```python
from build123d import *

# Parameters (mm, degrees)
F0_R     = 5.334
F0_R_2   = 1.778
F1_DEPTH = 3.81
F2_R     = 3.048
F3_DEPTH = 3.302


with BuildPart() as f1:
    # F0 (on Top) → F1 (new body)
    with BuildSketch(Plane.XY):
        Circle(F0_R)
        Circle(F0_R_2, mode=Mode.SUBTRACT)
        Circle(F0_R_2)
    extrude(amount=F1_DEPTH)

    # F2
    f2_edges = [f1.edges().sort_by_distance(p)[0] for p in [
        (-5.334, 0, 3.81),
    ]]
    fillet(f2_edges, radius=F2_R)

    # F0 (on Top) → F3 (cut)
    with BuildSketch(Plane.XY):
        Circle(F0_R_2)
    extrude(amount=F3_DEPTH, mode=Mode.SUBTRACT)


solid = f1.part
```
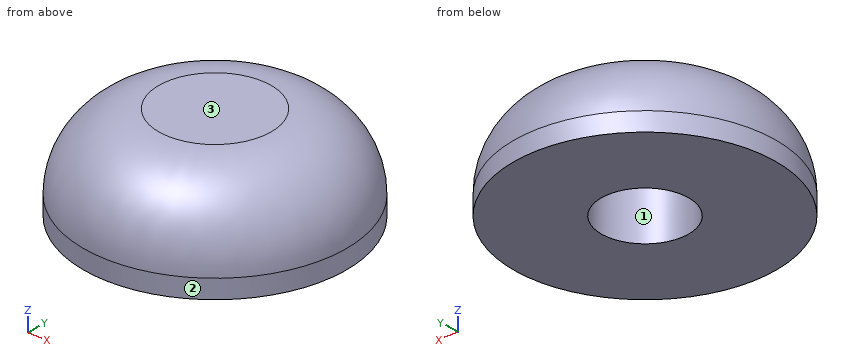
Geometry: final body of the model. Coordinates: model frame, mm. Face numbers are marked on the shaded views. Round coordinates to 2 decimals unless told otherwise and drop trailing zeros.
Item 1: Material intervals for L1, parallel to Z at x = 0.75, y = -1; L2, parallel to X at y = 1, z = 2.4; L3, parallel to Y at x = 0, z = 2.5, sorted ascending.
Item 2: Mould query, pull axis X, two halves, no side actions, for the marked faces 1, 2 and 3. Classes: +X half, -X half, draft (parallel to the pull), parting line (faces both ways), or undercut.
Item 3: Pin query (flat end, axial travel): P1, Ø1.5, axis at x = -1.5, z = 1.5, coming from the -Y side; P2, Ø1.1, axis at x = -1, y = -0.5, coming from the -Z side; P3, Ø1, axis at x = -3.5, y = -1, coming from the -Z side. Return the tip coordinate at first contact, or that it passes through.
Completed:
1. L1: z = 3.3 to 3.81
1. L2: x = -4.75 to -1.47, 1.47 to 4.75
1. L3: y = -4.79 to -1.78, 1.78 to 4.79
2. face 1: undercut
2. face 2: parting line
2. face 3: draft
3. P1: stops at y = -5.24
3. P2: stops at z = 3.3
3. P3: stops at z = 0
